```python
from build123d import *

# Parameters (mm, degrees)
SKETCH_1_W          = 18
SKETCH_1_H          = 130
SKETCH_1_W_2        = 5
SKETCH_1_H_2        = 2
SKETCH_1_H_3        = 3
EXTRUDE_1_DEPTH     = 1.05
SKETCH_5_R          = 0.5
CUT_EXTRUDE_3_DEPTH = 69.625141166
SKETCH_2_W          = 1.05
SKETCH_2_H          = 25.1
CUT_EXTRUDE_1_DEPTH = 10
SKETCH_6_R          = 0.5
CUT_EXTRUDE_4_DEPTH = 69.625141166
CUT_EXTRUDE_5_DEPTH = 69.625141166
CUT_EXTRUDE_6_DEPTH = 69.625141166
EXTRUDE_2_DEPTH     = 2.1
CUT_EXTRUDE_7_DEPTH = 72.731513298
FILLET_1_R          = 0.2
FILLET_2_R          = 1.5
FILLET_3_R          = 0.2


with BuildPart() as part:
    # 草图1 → 凸台-拉伸1 (new, symmetric)
    with BuildSketch(Plane.XY):
        Rectangle(SKETCH_1_W, SKETCH_1_H)
        with Locations((-2.5, 66)):
            Rectangle(SKETCH_1_W_2, SKETCH_1_H_2)
        with Locations((2.5, 66)):
            Rectangle(SKETCH_1_W_2, SKETCH_1_H_2)
        with Locations((2.5, -66.5)):
            Rectangle(SKETCH_1_W_2, SKETCH_1_H_3)
        with Locations((-2.5, -66.5)):
            Rectangle(SKETCH_1_W_2, SKETCH_1_H_3)
    extrude(amount=EXTRUDE_1_DEPTH, both=True)

    # 草图5 → 切除-拉伸3 (cut, through all)
    with BuildSketch(Plane.XY.offset(1.05)):
        with Locations((5.353553391, 65.353553391)):
            Circle(SKETCH_5_R)
        with Locations((-5.353553391, 65.353553391)):
            Circle(SKETCH_5_R)
        with Locations((5.353553391, -65.353553391)):
            Circle(SKETCH_5_R)
        with Locations((-5.353553391, -65.353553391)):
            Circle(SKETCH_5_R)
    extrude(amount=-CUT_EXTRUDE_3_DEPTH, mode=Mode.SUBTRACT)

    # 草图2 → 切除-拉伸1 (cut)
    with BuildSketch(Plane.XY.offset(1.05)):
        with Locations((0.525, 37.5)):
            Rectangle(SKETCH_2_W, SKETCH_2_H)
        with Locations((-0.525, 37.5)):
            Rectangle(SKETCH_2_W, SKETCH_2_H)
        with Locations((0.525, -37.5)):
            Rectangle(SKETCH_2_W, SKETCH_2_H)
        with Locations((-0.525, -37.5)):
            Rectangle(SKETCH_2_W, SKETCH_2_H)
    extrude(amount=-CUT_EXTRUDE_1_DEPTH, mode=Mode.SUBTRACT)

    # 草图6 → 切除-拉伸4 (cut, through all)
    with BuildSketch(Plane.XY.offset(1.05)):
        with Locations((0.696446609, 49.696446609)):
            Circle(SKETCH_6_R)
        with Locations((-0.696446609, 49.696446609)):
            Circle(SKETCH_6_R)
        with Locations((0.696446609, 25.303553391)):
            Circle(SKETCH_6_R)
        with Locations((-0.696446609, 25.303553391)):
            Circle(SKETCH_6_R)
    cut_extrude_4 = extrude(amount=-CUT_EXTRUDE_4_DEPTH, mode=Mode.SUBTRACT)

    # 镜向1: 切除-拉伸4 across plane
    add(cut_extrude_4.mirror(Plane.ZX), mode=Mode.SUBTRACT)

    # 草图4 → 切除-拉伸5 (cut, through all)
    with BuildSketch(Plane.XY.offset(1.05)):
        with BuildLine():
            Line((6.2, 55), (6.2, 35))
            ThreePointArc((6.2, 35), (5, 33.8), (3.8, 35))
            Line((3.8, 35), (3.8, 55))
            ThreePointArc((3.8, 55), (5, 56.2), (6.2, 55))
        make_face()
        with BuildLine():
            Line((6.2, 25), (6.2, 5))
            ThreePointArc((6.2, 5), (5, 3.8), (3.8, 5))
            Line((3.8, 5), (3.8, 25))
            ThreePointArc((3.8, 25), (5, 26.2), (6.2, 25))
        make_face()
        with BuildLine():
            Line((6.2, -5), (6.2, -25))
            ThreePointArc((6.2, -25), (5, -26.2), (3.8, -25))
            Line((3.8, -25), (3.8, -5))
            ThreePointArc((3.8, -5), (5, -3.8), (6.2, -5))
        make_face()
        with BuildLine():
            Line((3.8, -55), (3.8, -35))
            ThreePointArc((3.8, -35), (5, -33.8), (6.2, -35))
            Line((6.2, -35), (6.2, -55))
            ThreePointArc((6.2, -55), (5, -56.2), (3.8, -55))
        make_face()
    cut_extrude_5 = extrude(amount=-CUT_EXTRUDE_5_DEPTH, mode=Mode.SUBTRACT)

    # 镜向2: 切除-拉伸5 across plane
    add(cut_extrude_5.mirror(Plane(origin=(0, 0, 0), x_dir=(0, 0, 1), z_dir=(1, 0, 0))), mode=Mode.SUBTRACT)

    # 草图7 → 切除-拉伸6 (cut, through all)
    with BuildSketch(Plane.XY.offset(1.05)):
        with BuildLine():
            Line((1.2, 62.05), (1.2, 55.05))
            ThreePointArc((1.2, 55.05), (0, 53.85), (-1.2, 55.05))
            Line((-1.2, 55.05), (-1.2, 62.05))
            ThreePointArc((-1.2, 62.05), (0, 63.25), (1.2, 62.05))
        make_face()
        with BuildLine():
            Line((1.2, 15), (1.2, -15))
            ThreePointArc((1.2, -15), (0, -16.2), (-1.2, -15))
            Line((-1.2, -15), (-1.2, 15))
            ThreePointArc((-1.2, 15), (0, 16.2), (1.2, 15))
        make_face()
        with BuildLine():
            Line((1.2, -55.05), (1.2, -62.05))
            ThreePointArc((1.2, -62.05), (0, -63.25), (-1.2, -62.05))
            Line((-1.2, -62.05), (-1.2, -55.05))
            ThreePointArc((-1.2, -55.05), (0, -53.85), (1.2, -55.05))
        make_face()
    extrude(amount=-CUT_EXTRUDE_6_DEPTH, mode=Mode.SUBTRACT)

    # 草图8 → 凸台-拉伸2 (add)
    with BuildSketch(Plane.XY.offset(1.05)):
        Polygon((5, -68), (10, -68), (10, -71), (-10, -71), (-10, -68), (-5, -68), align=None)
        Polygon((5, 67), (10, 67), (10, 70), (-10, 70), (-10, 67), (-5, 67), align=None)
    extrude(amount=-EXTRUDE_2_DEPTH)

    # 草图9 → 切除-拉伸7 (cut, through all)
    with BuildSketch(Plane(origin=(0, 0, -1.05), x_dir=(-1, 0, 0), z_dir=(0, 0, -1))):
        with BuildLine():
            ThreePointArc((-4.853553391, -67.646446609), (-4.891613624, -67.455104893), (-5, -67.292893219))
            Line((-5, -67.292893219), (-5, -68))
            ThreePointArc((-5, -68), (-4.891613624, -67.837788326), (-4.853553391, -67.646446609))
        make_face()
        with BuildLine():
            ThreePointArc((-5.707106781, -68), (-5.353553391, -68.146446609), (-5, -68))
            Line((-5, -68), (-5.707106781, -68))
        make_face()
        with BuildLine():
            ThreePointArc((5, -67.292893219), (4.853553391, -67.646446609), (5, -68))
            Line((5, -68), (5, -67.292893219))
        make_face()
        with BuildLine():
            ThreePointArc((5, -68), (5.353553391, -68.146446609), (5.707106781, -68))
            Line((5.707106781, -68), (5, -68))
        make_face()
        with BuildLine():
            Line((5, 67), (5.707106781, 67))
            ThreePointArc((5.707106781, 67), (5.353553391, 67.146446609), (5, 67))
        make_face()
        with BuildLine():
            Line((5, 66.292893219), (5, 67))
            ThreePointArc((5, 67), (4.853553391, 66.646446609), (5, 66.292893219))
        make_face()
        with BuildLine():
            Line((-5, 67), (-5, 66.292893219))
            ThreePointArc((-5, 66.292893219), (-4.891613624, 66.455104893), (-4.853553391, 66.646446609))
            ThreePointArc((-4.853553391, 66.646446609), (-4.891613624, 66.837788326), (-5, 67))
        make_face()
        with BuildLine():
            Line((-5.707106781, 67), (-5, 67))
            ThreePointArc((-5, 67), (-5.353553391, 67.146446609), (-5.707106781, 67))
        make_face()
    extrude(amount=-CUT_EXTRUDE_7_DEPTH, mode=Mode.SUBTRACT)

    # 圆角1
    fillet_1_edges = [part.edges().sort_by_distance(p)[0] for p in [
        (5.707106781, 67, 0),
        (-5.707106781, 67, 0),
        (-5.707106781, -68, 0),
        (5, -67.292893219, 0),
        (5.707106781, -68, 0),
        (-5, -67.292893219, 0),
        (-5.707106781, -65, 0),
        (-5, -65.707106781, 0),
        (5, -65.707106781, 0),
        (5.707106781, -65, 0),
        (5.707106781, 65, 0),
        (-5.707106781, 65, 0),
    ]]
    fillet(fillet_1_edges, radius=FILLET_1_R)

    # 圆角2
    fillet_2_edges = [part.edges().sort_by_distance(p)[0] for p in [
        (10, -71, 0),
        (-10, -71, 0),
        (-10, 70, 0),
        (10, 70, 0),
    ]]
    fillet(fillet_2_edges, radius=FILLET_2_R)

    # 圆角3
    fillet_3_edges = [part.edges().sort_by_distance(p)[0] for p in [
        (-5, 66.292893219, 0),
        (5, 66.292893219, 0),
        (5, 65.707106781, 0),
        (-5, 65.707106781, 0),
    ]]
    fillet(fillet_3_edges, radius=FILLET_3_R)


solid = part.part
```
Geometry check sheet. Reference: the model listing, model coordinates, mm. Coordinates: 2 decimals unless noted, no trailing zeros. Order: outer loops, then holes, each group sorted by start corner. A loop starts at its lowest first (then second) coordinate and runs counter-clockwise, first axis right, second up. Notation, with made-up numbers: (-8.5, -29) - (22.5, -29) arc R28 ccw to (22.5, -11) - close; hole circle Ø11 at (67, -34). An arc over 180 degrees is marked (long way). Answer as a JSON object with one key per item and string values. Group by question number.
Item 1: Sectioned sample at A-A, the plane y = 30.5. Record the cut outline in (x, z).
Item 2: Sectioned sample at B-B, the plane y = -42. Record the cut outline in (x, z).
Item 3: Depth check by flat-ended pin: pin 1 Ø1 at (y, z) = (-49.5, -0.5) entering from -X; pin 2 Ø0.5 at (y, z) = (66, 0) entering from -X; pin 3 Ø0.6 at (y, z) = (-44, 0) entering from +X. Enter the tip coordinate at first touch or a pass-through.
Item 4: Sectioned sample at C-C, the plane z = -0.65. Give the number of separate pieces and of enclosed holes in the cut face, and give its area (3 significant figures).
Item 5: Scan lines: probe 1 along X at (y, z) = (35, 0.9); probe 2 along Y at (x, z) = (8.5, 0.9); probe 3 along Y at (x, z) = (0, -0.35). Record each from-to range of solid material in increasing order.
Resolved:
{
 "1": {"outline": "(-9, -1.05) - (-1.05, -1.05) - (-1.05, 1.05) - (-9, 1.05) - close; (1.05, -1.05) - (9, -1.05) - (9, 1.05) - (1.05, 1.05) - close"},
 "2": {"outline": "(-9, -1.05) - (-6.2, -1.05) - (-6.2, 1.05) - (-9, 1.05) - close; (-3.8, -1.05) - (-1.05, -1.05) - (-1.05, 1.05) - (-3.8, 1.05) - close; (1.05, -1.05) - (3.8, -1.05) - (3.8, 1.05) - (1.05, 1.05) - close; (6.2, -1.05) - (9, -1.05) - (9, 1.05) - (6.2, 1.05) - close"},
 "3": {"pin 1": "x = -9", "pin 2": "x = -5", "pin 3": "x = 9"},
 "4": {"separate pieces": "1", "enclosed holes": "13", "area": "1,860 mm^2"},
 "5": {"probe 1": "-9 to -6.2, -3.8 to -1.05, 1.05 to 3.8, 6.2 to 9", "probe 2": "-71 to -68, -65 to 65, 67 to 70", "probe 3": "-71 to -63.25, -53.85 to -50.05, -24.95 to -16.2, 16.2 to 24.95, 50.05 to 53.85, 63.25 to 70"}
}
